Can you work these out from the model? Positions are in its coordinate system, mm. A direction names the side the tool comes from. Coordinates: 2 decimals unless noted, no trailing zeros. Loops run counter-clockwise (first coordinate to the right, second up) from the corner with the lowest first, then second, coordinate; pieces in that order, holes last.
```python
from build123d import *

# Parameters (mm, degrees)
AUFSATZ_LINEAR_AUSTRAGEN1_DEPTH = 5
SKIZZE2_R                       = 50
SCHNITT_LINEAR_AUSTRAGEN1_DEPTH = 384.666521865
SKIZZE3_R                       = 3.5
AUFSATZ_LINEAR_AUSTRAGEN2_DEPTH = 4
FASE1_SIZE                      = 0.8
SCHNITT_LINEAR_AUSTRAGEN2_DEPTH = 384.666521865


with BuildPart() as part:
    # Skizze1 → Aufsatz-Linear austragen1 (new body)
    with BuildSketch(Plane(origin=(0, 0, 0), x_dir=(1, 0, 0), z_dir=(0, 1, 0))):
        with BuildLine():
            Line((150, 0), (290, 0))
            ThreePointArc((290, 0), (251.147367097, 145), (145, 251.147367097))
            Line((145, 251.147367097), (75, 129.903810568))
            ThreePointArc((75, 129.903810568), (129.903810568, 75), (150, 0))
        make_face()
    extrude(amount=AUFSATZ_LINEAR_AUSTRAGEN1_DEPTH)

    # Skizze2 → Schnitt-Linear austragen1 (cut, through all)
    with BuildSketch(Plane(origin=(0, 5, 0), x_dir=(1, 0, 0), z_dir=(0, 1, 0))):
        with Locations((112.5, 194.855715851)):
            Circle(SKIZZE2_R)
        with Locations(Location((194.855715851, 112.5, 0), (0, 0, 270))):
            Circle(SKIZZE2_R)
        with Locations((225, 0)):
            Circle(SKIZZE2_R)
    extrude(amount=-SCHNITT_LINEAR_AUSTRAGEN1_DEPTH, mode=Mode.SUBTRACT)

    # Skizze3 → Aufsatz-Linear austragen2 (add)
    with BuildSketch(Plane(origin=(0, 5, 0), x_dir=(1, 0, 0), z_dir=(0, 1, 0))):
        with Locations(Location((168.545626434, 22.189452677, 0), (0, 0, 270))):
            Circle(SKIZZE3_R)
        with Locations(Location((277.604561185, 36.547333822, 0), (0, 0, 270))):
            Circle(SKIZZE3_R)
        with Locations(Location((157.059520527, 65.056183502, 0), (0, 0, 270))):
            Circle(SKIZZE3_R)
        with Locations(Location((134.87006785, 103.489442931, 0), (0, 0, 270))):
            Circle(SKIZZE3_R)
        with Locations(Location((103.489442931, 134.87006785, 0), (0, 0, 270))):
            Circle(SKIZZE3_R)
        with Locations(Location((170.453200122, 222.138935282, 0), (0, 0, 270))):
            Circle(SKIZZE3_R)
        with Locations(Location((222.138935282, 170.453200122, 0), (0, 0, 270))):
            Circle(SKIZZE3_R)
        with Locations(Location((258.686269103, 107.151361062, 0), (0, 0, 270))):
            Circle(SKIZZE3_R)
    extrude(amount=AUFSATZ_LINEAR_AUSTRAGEN2_DEPTH)

    # Fase1
    fase1_edges = [part.edges().sort_by_distance(p)[0] for p in [
        (168.545626434, 9, -25.689452677),
        (277.604561185, 9, -40.047333822),
        (157.059520527, 9, -68.556183502),
        (134.87006785, 9, -106.989442931),
        (103.489442931, 9, -138.37006785),
        (170.453200122, 9, -225.638935282),
        (222.138935282, 9, -173.953200122),
        (258.686269103, 9, -110.651361062),
    ]]
    chamfer(fase1_edges, length=FASE1_SIZE)

    # Skizze4 → Schnitt-Linear austragen2 (cut, through all)
    with BuildSketch(Plane(origin=(0, 5, 0), x_dir=(1, 0, 0), z_dir=(0, 1, 0))):
        with BuildLine():
            Line((100.63005083, 111.236652548), (111.369318037, 121.975919755))
            Line((111.369318037, 121.975919755), (121.975919755, 111.369318037))
            Line((121.975919755, 111.369318037), (111.236652548, 100.63005083))
            ThreePointArc((111.236652548, 100.63005083), (106.066017178, 106.066017178), (100.63005083, 111.236652548))
        make_face()
        with BuildLine():
            Line((142.766506677, 46.018741523), (157.436618499, 49.949586139))
            Line((157.436618499, 49.949586139), (161.318904176, 35.460698745))
            Line((161.318904176, 35.460698745), (146.648792353, 31.529854129))
            ThreePointArc((146.648792353, 31.529854129), (144.888873943, 38.822856765), (142.766506677, 46.018741523))
        make_face()
    extrude(amount=-SCHNITT_LINEAR_AUSTRAGEN2_DEPTH, mode=Mode.SUBTRACT)


solid = part.part
```
Item 1: Suppose I cut it at B-B, the plane z = -210. Please give me the cut outline in (x, y), plus the area to 3 significant figures.
Results are:
outline: (160.15, 0) - (200, 0) - (200, 5) - (160.15, 5) - close
area: 199 mm2
Item 2: We'd pull the mould along X, two halves only. Please class faces 3 (the face through (105.855, 6.578, -137.45)), 4 (the face through (129.681, 2.465, -75.385)), 5 (the face through (116.598, 2.535, -116.747)), 6 (the face through (159.35, 2.54, -42.81)): +X half, -X half, draft (parallel to the pull), parting line (faces both ways), or undercut.
Results are:
face 3: parting line
face 4: -X half
face 5: undercut
face 6: undercut
Item 3: I'm going to push flat-ended pins straight in: P1, Ø3, axis at x = 218.5, y = 6, coming from the -Z side; P2, Ø1, axis at y = 4.5, z = -68, coming from the -X side; P3, Ø5, axis at x = 199.5, y = 3, coming from the -Z side. Where does each tip first touch, or does it pass through?
Results are:
P1: stops at z = -191.95
P2: stops at x = 133.45
P3: stops at z = -212.82
Item 4: On a 3-axis mill with a long thin cutter (end or side, diameter ignored), from which of +Z, -Z, +X, -X, +Y, -Y can I reach the whole of each face in a straight line? I mean faces 1 (the face through (150, 0, -89)), 2 (the face through (154.93, 6.578, -67.834)). Say none if no direction works.
Results are:
face 1: +Z, -Z, +X, -X, -Y
face 2: +Y
Item 5: Suppose I cut it at A-A, the plane y = 6.5. Please give me the cut outline in (x, z), plus the area to 3 significant figures.
Results are:
outline: circle Ø7 at (103.49, -134.87); circle Ø7 at (134.87, -103.49); circle Ø7 at (157.06, -65.06); circle Ø7 at (168.55, -22.19); circle Ø7 at (170.45, -222.14); circle Ø7 at (222.14, -170.45); circle Ø7 at (258.69, -107.15); circle Ø7 at (277.6, -36.55)
area: 308 mm2
Item 6: I need wall thicknesses on line 1 along X through (y, z) = (3.5, -112.5); line 2 along X through (y, z) = (3, -27); line 3 along Y through (x, z) = (188.5, -170). Which ranges of each line are inside material? Lowest first, please.
Results are:
line 1: x = 99.22 to 101.89, 120.85 to 144.86, 244.86 to 267.29
line 2: x = 147.55 to 182.92, 267.08 to 288.74
line 3: y = 0 to 5
